Part model, mm, in its own coordinate system. A direction names the side the tool comes from. Round coordinates to 2 decimals unless told otherwise and drop trailing zeros. Loops run counter-clockwise (first coordinate to the right, second up) from the corner with the lowest first, then second, coordinate; pieces in that order, holes last. Notation, with made-up numbers: M -9,73.25 L 7,73.25 A25 cw 7,97.25 Z; hole C -2,40.25 d9. An arc over 180 degrees is marked long. Answer as CSV lines item,"result". Start each with the question number.
Item 1: Which spindle directions (+Z, -Z, +X, -X, +Y, -Y) get a long thin tool onto all of the face, cutting with end or side? Do faces 1 (the flat face through (2, 10, 23)), 2 (the flat face through (1, 7.75, 2)), 3 (the cylindrical face through (2.46, 6.25, 24.47)), 4 (the flat face through (2, 1.75, 29)), 5 (the flat face through (2, 12.75, 16)). Say none if no direction does.
Item 2: Band-saw the part on D-D (x = 2.1). Give the cut face in (y, z).
Item 3: Band-saw the part on B-B (z = 7.5). Give the cut face in (x, y).
Item 4: Band-saw the part on A-A (x = 0.55). Give the cut face in (y, z).
Item 5: Band-saw the part on C-C (z = 3). Give the cut face in (x, y), and give its area (3 significant figures).
Item 6: Drop flat-ended pins along their axis: pin 1 Ø2 at (x, z) = (2, 26.5) entering from +Y; pin 2 Ø1.5 at (x, y) = (2.5, 4) entering from -Z; pin 3 Ø1.3 at (x, y) = (2, 10.5) entering from +Z. Give the stop position or say it passes through.
Item 7: Mould opens along X. For faces 6 (the cylindrical face through (1.669, 4.708, 28.094)), 7 (the cylindrical face through (2.54, -6.85, 31.14)), 8 (the flat face through (0, 0, 14)) say: pulls with the +X half, pulls with the -X half, needs draft (parallel to the pull), parting line crosses it, or undercut.
Item 8: Wall check: line 1 (X direction, y = 3.25, z = 3); line 2 (Z direction, x = 2.5, y = 3.35); line 3 (Z direction, x = 4.3, y = -0.25). Give the ranges that are in metal, low to high.
Autodesk Inventor part; units mm, degrees
ref_plane "YZ Plane" through (0, 0, 0) normal (1, 0, 0) x (0, 1, 0)
ref_plane "XZ Plane" through (0, 0, 0) normal (0, 1, 0) x (-1, 0, 0)
ref_plane "XY Plane" through (0, 0, 0) normal (0, 0, 1) x (1, 0, 0)
sketch "Sketch1" plane through (0, 0, 0) normal (1, 0, 0) x (0, 1, 0)
  line L0 (0.25, 0) -> (0.25, -5)
  line L1 (0.25, -5) -> (-7.75, -5)
  line L2 (-7.75, -5) -> (-7.75, 32)
  line L3 (-7.75, 32) -> (7.75, 32)
  line L4 (7.75, 32) -> (7.75, 23)
  line L5 (7.75, 23) -> (12.75, 23)
  line L6 (12.75, 23) -> (12.75, 9)
  line L7 (12.75, 9) -> (7.75, 9)
  line L8 (0.25, 0) -> (7.75, 0)
  line L9 (7.75, 0) -> (7.75, 9)
  line L10 (0, -5) -> (0, 32) construction
  line L11 (12.75, 16) -> (-7.75, 16) construction
  arc A0 (7.75, 26) -> (7.75, 23) centre (7.75, 24.5) ccw
  arc A1 (7.75, 9) -> (7.75, 6) centre (7.75, 7.5) ccw
  arc A2 (2.3713, 0) -> (0.25, -2.1213) centre (1.3107, -1.0607) ccw
  line L12 (7.75, 29) -> (1.75, 29) construction
  line L13 (7.75, 3) -> (1.75, 3) construction
  point P0 (0, 0)
  point P1 (0, 25)
  point P2 (0, 7)
  point P3 (7.75, 6)
  point P4 (4.1709, -1.359)
  point P5 (4.291, 0)
  dimension "d6" = 5
  dimension "d7" = 14
  dimension "d8" = 5
  dimension "d9" = 18
  dimension "d12" = 6
  dimension "d13" = 6
  dimension "d31" = 9
  dimension "d32" = 1.5
  dimension "d33" = 32
  dimension "d34" = 8
  dimension "d35" = 15.5
extrude "Extrusion1" add sketch "Sketch1" along normal blind 5 contours A2 L0 L1 L2 L3 L4 A0 L5 L6 L7 A1 L9 L8
sketch "Sketch2" plane through (0, 7.75, 32) normal (0, 1, 0) x (1, 0, 0)
  line L0 (5, 3) -> (0, 3)
  line L1 (0, 9) -> (0, 0)
  line L2 (5, 32) -> (5, 23)
  line L3 (5, 29) -> (0, 29)
  line L4 (5, 9) -> (5, 0)
  point P0 (0, 32)
  point P1 (0, 6)
  point P2 (5, 26)
  point P3 (5, 6)
  point P4 (0, 29)
  point P5 (0, 29)
  point P6 (0, 29)
  point P7 (2.5, 29)
  point P8 (2.5, 3)
hole "Hole1" at (2.5, 7.75, 3) at (2.5, 7.75, 29) direction (0, -1, 0) diameter 2.459 depth 6
hole "Hole2" at (0, 0, 25) at (0, 0, 7) direction (1, 0, 0) diameter 2.459 end through all
chamfer "Chamfer1" distance 0.5 angle 45 4 edges at (2.5, -7.75, -5) (2.5, 0.25, -5) (2.5, 12.75, 9) (2.5, 12.75, 23)
fillet "Fillet1" radius 3 1 edges at (2.5, -7.75, 32)
properties part number "TorsoAngleBraceFrame" material "Acetal Resin, Black"
Answer block:
1,face 1,"+Z, +X, -X, +Y"
1,face 2,"-Z, +X, -X, +Y"
1,face 3,"+X, -X, +Y"
1,face 4,"+Y"
1,face 5,"+Z, -Z, +X, -X, +Y"
2,outline,"M -7.75,-4.5 L -7.25,-5 L -0.25,-5 L 0.25,-4.5 L 0.25,-2.12 A1.5 cw 2.37,0 L 7.75,0 L 7.75,1.84 L 1.75,1.84 L 1.75,4.16 L 7.75,4.16 L 7.75,6 A1.5 cw 7.75,9 L 12.25,9 L 12.75,9.5 L 12.75,22.5 L 12.25,23 L 7.75,23 A1.5 cw 7.75,26 L 7.75,27.84 L 1.75,27.84 L 1.75,30.16 L 7.75,30.16 L 7.75,32 L -4.75,32 A3 ccw -7.75,29 Z; hole C 0,7 d2.46; hole C 0,25 d2.46"
3,outline,"M 0,-7.75 L 5,-7.75 L 5,-1.12 L 0,-1.12 Z; M 0,1.12 L 5,1.12 L 5,6.25 L 0,6.25 Z"
4,outline,"M -7.75,-4.5 L -7.25,-5 L -0.25,-5 L 0.25,-4.5 L 0.25,-2.12 A1.5 cw 2.37,0 L 7.75,0 L 7.75,6 A1.5 cw 7.75,9 L 12.25,9 L 12.75,9.5 L 12.75,22.5 L 12.25,23 L 7.75,23 A1.5 cw 7.75,26 L 7.75,32 L -4.75,32 A3 ccw -7.75,29 Z; hole C 0,7 d2.46; hole C 0,25 d2.46"
5,outline,"M 0,-7.75 L 5,-7.75 L 5,7.75 L 3.73,7.75 L 3.73,1.75 L 1.27,1.75 L 1.27,7.75 L 0,7.75 Z"
5,area,"62.7 mm^2"
6,pin 1,"stops at y = 7.75"
6,pin 2,"stops at z = 0"
6,pin 3,"stops at z = 23"
7,face 6,"undercut"
7,face 7,"needs draft"
7,face 8,"pulls with the -X half"
8,line 1,"x = 0 to 1.27, 3.73 to 5"
8,line 2,"z = 0 to 1.77, 4.23 to 27.77, 30.23 to 32"
8,line 3,"z = -5 to 5.8, 8.2 to 23.8, 26.2 to 32"
